For this review, take the finished solid that the model builds, in its own axes (mm). Face numbers are marked on the shaded views. Coordinates: 2 decimals unless noted, no trailing zeros. Loops run counter-clockwise (first coordinate to the right, second up) from the corner with the lowest first, then second, coordinate; pieces in that order, holes last.
1. Take a section at B-B, the plane z = 0. State the section outline as (x, y) points, then the cut area to 3 significant figures.
2. Mouldability with a two-part tool opening along X and no side actions: class the marked faces 1, 2 and 3 as pulls with the +X half, pulls with the -X half, needs draft (parallel to the pull), parting line crosses it, or undercut.
3. Take a section at A-A, the plane x = 0. State the section outline as (y, z) points, then the cut area to 3 significant figures.
4. To check wall thickness, follow probe 1 along Y at (x, z) = (9, 13); probe 2 along X at (y, z) = (-5.25, 0); probe 3 along Z at (x, y) = (1.5, -18.25). State the ranges of each line that lie inside material, in increasing order.
5. Take a section at D-D, the plane y = -6.75. State the section outline as (x, z) points, then the cut area to 3 significant figures.
6. Clearance check with flat-ended pins moving along their axes: P1, Ø10, axis at x = -16.5, y = -21, coming from the +Z side; P2, Ø3, axis at y = -19.5, z = -10.5, coming from the +X side; P3, Ø2.5, axis at x = 20.62, z = 11.91, coming from the -Y side. State where each tip first meets the part, or that it passes through.
7. Take a section at C-C, the plane x = -19.5. State the section outline as (y, z) points.
```python
from build123d import *

# Parameters (mm, degrees)
SKETCH1_R           = 30.48
SKETCH1_R_2         = 2.15265
BOSS_EXTRUDE1_DEPTH = 2
CUT_EXTRUDE1_DEPTH  = 10
SKETCH3_R           = 13
SKETCH3_R_2         = 3.110414615
BOSS_EXTRUDE2_DEPTH = 25.4


with BuildPart() as part:
    # Sketch1 → Boss-Extrude1 (new body)
    with BuildSketch(Plane(origin=(0, 0, 0), x_dir=(1, 0, 0), z_dir=(0, 1, 0))):
        with Locations(Location((0, 0, 0), (0, 0, 270))):
            Circle(SKETCH1_R)
        with Locations(Location((0, -23.8125, 0), (0, 0, 270))):
            Circle(SKETCH1_R_2, mode=Mode.SUBTRACT)
        with Locations(Location((20.622229928, -11.90625, 0), (0, 0, 270))):
            Circle(SKETCH1_R_2, mode=Mode.SUBTRACT)
        with Locations(Location((20.622229928, 11.90625, 0), (0, 0, 270))):
            Circle(SKETCH1_R_2, mode=Mode.SUBTRACT)
        with Locations(Location((0, 23.8125, 0), (0, 0, 270))):
            Circle(SKETCH1_R_2, mode=Mode.SUBTRACT)
        with Locations(Location((-20.622229928, 11.90625, 0), (0, 0, 270))):
            Circle(SKETCH1_R_2, mode=Mode.SUBTRACT)
        with Locations(Location((-20.622229928, -11.90625, 0), (0, 0, 270))):
            Circle(SKETCH1_R_2, mode=Mode.SUBTRACT)
    extrude(amount=BOSS_EXTRUDE1_DEPTH)

    # Sketch2 → Cut-Extrude1 (cut)
    with BuildSketch(Plane(origin=(0, 2, 0), x_dir=(1, 0, 0), z_dir=(0, 1, 0))):
        with BuildLine():
            ThreePointArc((1.93204455, 2.295038966), (-2.879237228, -0.842610814), (2.864533851, -0.8913169))
            Line((2.864533851, -0.8913169), (1.93204455, 2.295038966))
        make_face()
    extrude(amount=-CUT_EXTRUDE1_DEPTH, mode=Mode.SUBTRACT)

    # Sketch3 → Boss-Extrude2 (add)
    # profile 1 of 2: a face of its own
    with BuildSketch(Plane.XZ):
        with Locations(Location((0, 0, 0), (0, 0, 90))):
            Circle(SKETCH3_R)
        Circle(SKETCH3_R_2, mode=Mode.SUBTRACT)
    # profile 2 of 2: a face of its own
    with BuildSketch(Plane.XZ):
        Circle(SKETCH3_R_2)
        with BuildLine():
            Line((2.864533851, 0.8913169), (1.93204455, -2.295038966))
            ThreePointArc((1.93204455, -2.295038966), (-2.879237228, 0.842610814), (2.864533851, 0.8913169))
        make_face(mode=Mode.SUBTRACT)
    extrude(amount=BOSS_EXTRUDE2_DEPTH)


solid = part.part
```
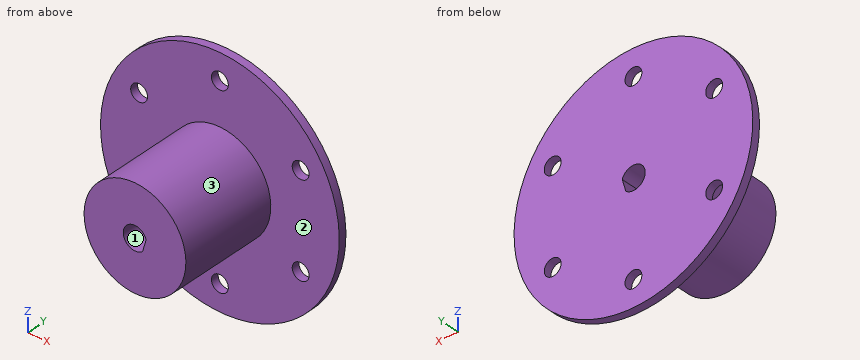
Results list:
1. outline: (-30.48, 0) - (-13, 0) - (-13, -25.4) - (-3, -25.4) - (-3, 2) - (-30.48, 2) - close; (2.6, -25.4) - (13, -25.4) - (13, 0) - (30.48, 0) - (30.48, 2) - (2.6, 2) - close
1. area: 629 mm2
2. face 1: undercut
2. face 2: needs draft
2. face 3: parting line crosses it
3. outline: (-25.4, -13) - (0, -13) - (0, -21.66) - (2, -21.66) - (2, -3) - (-25.4, -3) - close; (-25.4, 3) - (2, 3) - (2, 21.66) - (0, 21.66) - (0, 13) - (-25.4, 13) - close; (0, -30.48) - (2, -30.48) - (2, -25.97) - (0, -25.97) - close; (0, 25.97) - (2, 25.97) - (2, 30.48) - (0, 30.48) - close
3. area: 601 mm2
4. probe 1: y = 0 to 2
4. probe 2: x = -13 to -3, 2.6 to 13
4. probe 3: z = -12.91 to -2.6, 2.6 to 12.91
5. outline: circle Ø26 at (0, 0); hole (1.93, -2.3) - (2.86, 0.89) arc R3 ccw (long way) to start
5. area: 504 mm2
6. P1: stops at z = 6.06
6. P2: stops at x = 9.38
6. P3: passes through
7. outline: (0, -23.43) - (2, -23.43) - (2, -13.74) - (0, -13.74) - close; (0, -10.07) - (2, -10.07) - (2, 10.07) - (0, 10.07) - close; (0, 13.74) - (2, 13.74) - (2, 23.43) - (0, 23.43) - close
